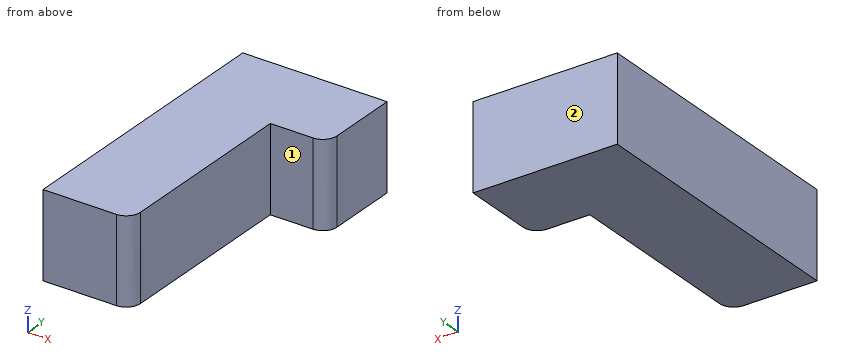
from build123d import *

# Parameters (mm, degrees)
BOSS_EXTRUDE1_DEPTH = 3
FILLET1_R           = 0.5
FILLET3_R           = 0.5


with BuildPart() as part:
    # Sketch1 → Boss-Extrude1 (new body)
    with BuildSketch(Plane.XY):
        Polygon((-6.445210562, 7.139162572), (-1.365210562, 7.139162572), (-1.365210562, 4.139162572), (-3.365210562, 4.139162572), (-3.365210562, -2.860837428), (-6.445210562, -2.860837428), align=None)
    extrude(amount=BOSS_EXTRUDE1_DEPTH)

    # Fillet1
    fillet1_edges = [part.edges().sort_by_distance(p)[0] for p in [
        (-3.365210562, -2.860837428, 1.5),
    ]]
    fillet(fillet1_edges, radius=FILLET1_R)

    # Fillet3
    fillet3_edges = [part.edges().sort_by_distance(p)[0] for p in [
        (-1.365210562, 4.139162572, 1.5),
    ]]
    fillet(fillet3_edges, radius=FILLET3_R)


solid = part.part
Verification items for the finished model (mm, model axes). Face numbers are marked on the shaded views. A direction names the side the tool comes from. Give positions to 0.01 mm unless a question says otherwise; leave off trailing zeros. Order: outer loops, then holes, each group sorted by start corner. A loop starts at its lowest first (then second) coordinate and runs counter-clockwise, first axis right, second up. Notation, with made-up numbers: M 19.25,19 L 61.25,19 A14 cw 61.25,35 Z; hole C -20.75,53.25 d3. An arc over 180 degrees is marked long. Answer as a JSON object with one key per item and string values. Group by question number.
1) Cross-section at C-C (x = -2.3). Enter the section's corners in (y, z).
2) Depth check by flat-ended pin: pin 1 Ø1 at (x, z) = (-2.5, 1) entering from -Y. Enter the tip coordinate at first touch or a pass-through.
3) Cross-section at B-B (y = -1.75). Enter the section's corners in (x, z).
4) Access from +Z, -Z, +X, -X, +Y, -Y to the whole of each face (thin tool, end or side, straight path). Record for the marked faces 1 and 2.
5) Scan lines: line 1 along X through (y, z) = (2.25, 1.6); line 2 along Y through (x, z) = (-2.9, 2.25); line 3 along X through (y, z) = (4.5, 2.55). Record each from-to range of solid material in increasing order. Write a range as [from, to].
6) Cross-section at A-A (z = 0.6). Enter the section's corners in (x, y).
Result sheet:
{
 "1": {"outline": "M 4.14,0 L 7.14,0 L 7.14,3 L 4.14,3 Z"},
 "2": {"pin 1": "stops at y = 4.14"},
 "3": {"outline": "M -6.45,0 L -3.37,0 L -3.37,3 L -6.45,3 Z"},
 "4": {"face 1": "+Z, -Z, +X, -Y", "face 2": "+Z, -Z, +X, -X, +Y"},
 "5": {"line 1": "x = [-6.45, -3.37]", "line 2": "y = [4.14, 7.14]", "line 3": "x = [-6.45, -1.38]"},
 "6": {"outline": "M -6.45,-2.86 L -3.87,-2.86 A0.5 ccw -3.37,-2.36 L -3.37,4.14 L -1.87,4.14 A0.5 ccw -1.37,4.64 L -1.37,7.14 L -6.45,7.14 Z"}
}
